Verification items for the finished model (mm, model axes). Face numbers are marked on the shaded views. A direction names the side the tool comes from. Coordinates: 2 decimals unless noted, no trailing zeros. Loops run counter-clockwise (first coordinate to the right, second up) from the corner with the lowest first, then second, coordinate; pieces in that order, holes last. Notation, with made-up numbers: (11, 23) -> (54, 23) arc R32 ccw to (54, 59) -> close; hole circle Ø4 at (74.5, -40). An arc over 180 degrees is marked (long way). Use CSV: the item, a comma, the result in double quotes. Start each with the question number.
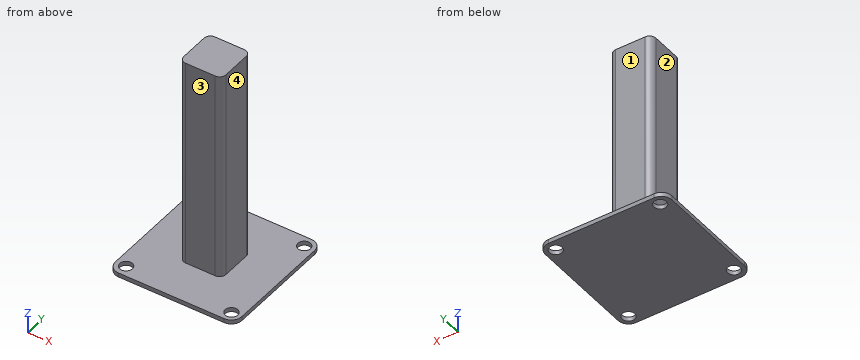
```python
from build123d import *

# Parameters (mm, degrees)
SKETCH_W     = 20
SKETCH_H     = 20
PAD_DEPTH    = 100
FILLET_R     = 3
FILLET001_R  = 3
SKETCH001_W  = 60
SKETCH001_H  = 60
PAD001_DEPTH = 2
FILLET002_R  = 5
FILLET003_R  = 5
FILLET004_R  = 5
FILLET005_R  = 5
SKETCH002_R  = 3
HOLE_DEPTH   = 25
HOLE_TIPS_R  = 3


with BuildPart() as part:
    # Sketch → Pad (new body)
    with BuildSketch(Plane.XY):
        with Locations((10, -10)):
            Rectangle(SKETCH_W, SKETCH_H)
    extrude(amount=PAD_DEPTH)

    # Fillet
    fillet_edges = [part.edges().sort_by_distance(p)[0] for p in [
        (0, -20, 50),
        (20, 0, 50),
        (0, 0, 50),
    ]]
    fillet(fillet_edges, radius=FILLET_R)

    # Fillet001
    fillet001_edges = [part.edges().sort_by_distance(p)[0] for p in [
        (20, -20, 50),
    ]]
    fillet(fillet001_edges, radius=FILLET001_R)

    # Sketch001 (on Face1 of Fillet001) → Pad001 (join)
    with BuildSketch(Plane(origin=(0, 0, 0), x_dir=(1, 0, 0), z_dir=(0, 0, -1))):
        with Locations((10, 10)):
            Rectangle(SKETCH001_W, SKETCH001_H)
    extrude(amount=PAD001_DEPTH)

    # Fillet002
    fillet002_edges = [part.edges().sort_by_distance(p)[0] for p in [
        (-20, 20, -1),
    ]]
    fillet(fillet002_edges, radius=FILLET002_R)

    # Fillet003
    fillet003_edges = [part.edges().sort_by_distance(p)[0] for p in [
        (40, 20, -1),
    ]]
    fillet(fillet003_edges, radius=FILLET003_R)

    # Fillet004
    fillet004_edges = [part.edges().sort_by_distance(p)[0] for p in [
        (-20, -40, -1),
    ]]
    fillet(fillet004_edges, radius=FILLET004_R)

    # Fillet005
    fillet005_edges = [part.edges().sort_by_distance(p)[0] for p in [
        (40, -40, -1),
    ]]
    fillet(fillet005_edges, radius=FILLET005_R)

    # Sketch002 (on Face18 of Fillet005) → Hole (cut)
    with BuildSketch(Plane(origin=(0, 0, -2), x_dir=(1, 0, 0), z_dir=(0, 0, -1))):
        with Locations((-14.665156, -15.297529)):
            Circle(SKETCH002_R)
        with Locations((35.039818, -15.044578)):
            Circle(SKETCH002_R)
        with Locations((35.166283, 35.166294)):
            Circle(SKETCH002_R)
        with Locations((-15.044579, 34.786861)):
            Circle(SKETCH002_R)
    extrude(amount=-HOLE_DEPTH, mode=Mode.SUBTRACT)

    # Hole tips → Hole tip 1 section 0
    with BuildSketch(Plane(origin=(0, 0, 23), x_dir=(1, 0, 0), z_dir=(0, 0, -1)), mode=Mode.PRIVATE) as hole_tip_1_s0:
        with Locations((-14.665156, -15.297529)):
            Circle(HOLE_TIPS_R)
    loft([hole_tip_1_s0.sketch, Vertex(-14.665156, 15.297529, 24.802582)], mode=Mode.SUBTRACT)

    # Hole tips → Hole tip 2 section 0
    with BuildSketch(Plane(origin=(0, 0, 23), x_dir=(1, 0, 0), z_dir=(0, 0, -1)), mode=Mode.PRIVATE) as hole_tip_2_s0:
        with Locations((35.039818, -15.044578)):
            Circle(HOLE_TIPS_R)
    loft([hole_tip_2_s0.sketch, Vertex(35.039818, 15.044578, 24.802582)], mode=Mode.SUBTRACT)

    # Hole tips → Hole tip 3 section 0
    with BuildSketch(Plane(origin=(0, 0, 23), x_dir=(1, 0, 0), z_dir=(0, 0, -1)), mode=Mode.PRIVATE) as hole_tip_3_s0:
        with Locations((35.166283, 35.166294)):
            Circle(HOLE_TIPS_R)
    loft([hole_tip_3_s0.sketch, Vertex(35.166283, -35.166294, 24.802582)], mode=Mode.SUBTRACT)

    # Hole tips → Hole tip 4 section 0
    with BuildSketch(Plane(origin=(0, 0, 23), x_dir=(1, 0, 0), z_dir=(0, 0, -1)), mode=Mode.PRIVATE) as hole_tip_4_s0:
        with Locations((-15.044579, 34.786861)):
            Circle(HOLE_TIPS_R)
    loft([hole_tip_4_s0.sketch, Vertex(-15.044579, -34.786861, 24.802582)], mode=Mode.SUBTRACT)


solid = part.part
```
1. Set-up check for the marked faces 1, 2, 3 and 4: record each of +Z, -Z, +X, -X, +Y, -Y from which the full face is reachable in a straight line by a thin tool's end or side.
2. Depth check by flat-ended pin: pin 1 (4 mm diameter, centred on x = 7.5, z = 32, fed in from +Y); pin 2 (8 mm diameter, centred on y = 7.5, z = 61, fed in from -X); pin 3 (15.5 mm diameter, centred on x = 9, z = 48.5, fed in from -Y); pin 4 (11 mm diameter, centred on y = -7.5, z = 25.5, fed in from -X). Enter the tip coordinate at first touch or a pass-through.
3. Cross-section at B-B, the plane y = -33.5. Record the boundary of the cut face in (x, z), plus the area to 3 significant figures.
4. Scan lines: line 1 (Y direction, x = 17, z = 75); line 2 (Z direction, x = 3.5, y = 8); line 3 (X direction, y = -8.5, z = 24.5). Record each from-to range of solid material in increasing order.
5. Cross-section at C-C, the plane x = 8. Record the boundary of the cut face in (y, z), plus the area to 3 significant figures.
6. Cross-section at A-A, the plane z = 46. Record the boundary of the cut face in (x, y).
7. Cross-section at D-D, the plane x = 21.5. Record the boundary of the cut face in (y, z).
Solution:
1,face 1,"+Z, +X, -X, +Y"
1,face 2,"+Z, -X, +Y, -Y"
1,face 3,"+Z, +X, -X, -Y"
1,face 4,"+Z, +X, +Y, -Y"
2,pin 1,"stops at y = 0"
2,pin 2,"passes through"
2,pin 3,"stops at y = -20"
2,pin 4,"stops at x = 0"
3,outline,"(-20, -2) -> (-17.75, -2) -> (-17.75, 0) -> (-20, 0) -> close; (-12.33, -2) -> (32.67, -2) -> (32.67, 0) -> (-12.33, 0) -> close; (37.66, -2) -> (40, -2) -> (40, 0) -> (37.66, 0) -> close"
3,area,"99.2 mm2"
4,line 1,"y = -20 to 0"
4,line 2,"z = -2 to 0"
4,line 3,"x = 0 to 20"
5,outline,"(-40, -2) -> (20, -2) -> (20, 0) -> (0, 0) -> (0, 100) -> (-20, 100) -> (-20, 0) -> (-40, 0) -> close"
5,area,"2,120 mm2"
6,outline,"(0, -17) arc R3 ccw to (3, -20) -> (17, -20) arc R3 ccw to (20, -17) -> (20, -3) arc R3 ccw to (17, 0) -> (3, 0) arc R3 ccw to (0, -3) -> close"
7,outline,"(-40, -2) -> (20, -2) -> (20, 0) -> (-40, 0) -> close"
